Autodesk Inventor part; units mm, degrees
ref_plane "Work Plane1" through (-97.3094, -87.3563, -6.35) normal (0, 0, -1) x (0, 1, 0)
ref_plane "YZ Plane" through (0, 0, 0) normal (1, 0, 0) x (0, 1, 0)
ref_plane "XZ Plane" through (0, 0, 0) normal (0, 1, 0) x (-1, 0, 0)
sketch "Sketch1" plane through (0, 0, 0) normal (0, 0, 1) x (1, 0, 0)
  line L0 (-65.7194, 60.3542) -> (-75.7574, -47.1434)
  line L1 (-75.7574, -47.1434) -> (65.7194, -60.3542)
  line L2 (-95.8276, -262.0778) -> (45.6492, -275.2887)
  line L3 (-105.8656, -369.5754) -> (-95.8276, -262.0778)
  line L4 (-212.6955, 74.0786) -> (-222.7334, -33.419)
  line L5 (-222.7334, -33.419) -> (-364.2102, -20.2081)
  line L6 (-242.8036, -248.3534) -> (-384.2805, -235.1426)
  line L7 (-252.8416, -355.851) -> (-242.8036, -248.3534)
  circle A0 centre (-72.4386, -92.2695) radius 2.6 construction
  circle A1 centre (-84.3392, -219.7151) radius 2.6 construction
  circle A2 centre (3.2796, -227.8968) radius 2.6 construction
  circle A3 centre (15.1803, -100.4512) radius 2.6 construction
  circle A4 centre (-156.3158, -105.5656) radius 1.7526 construction
  circle A5 centre (-164.2553, -190.5905) radius 1.7526 construction
  circle A6 centre (-246.2503, -204.5961) radius 2.6 construction
  circle A7 centre (-333.8691, -196.4144) radius 2.6 construction
  circle A8 centre (-321.9685, -68.9688) radius 2.6 construction
  circle A9 centre (-234.3496, -77.1505) radius 2.6 construction
  circle A10 centre (15.1803, -100.4512) radius 1.6
  circle A11 centre (3.2796, -227.8968) radius 1.6
  circle A12 centre (-84.3392, -219.7151) radius 1.6
  circle A13 centre (-72.4386, -92.2695) radius 1.6
  circle A14 centre (-234.3496, -77.1505) radius 1.6
  circle A15 centre (-321.9685, -68.9688) radius 1.6
  circle A16 centre (-333.8691, -196.4144) radius 1.6
  circle A17 centre (-246.2503, -204.5961) radius 1.6
  line L8 (-65.7194, 60.3542) -> (-212.6955, 74.0786)
  line L9 (-364.2102, -20.2081) -> (-384.2805, -235.1426)
  line L10 (-252.8416, -355.851) -> (-105.8656, -369.5754)
  line L11 (45.6492, -275.2887) -> (65.7194, -60.3542)
  circle A18 centre (-156.3158, -105.5656) radius 1.8288
  circle A19 centre (-164.2553, -190.5905) radius 1.8288
  point P0 (0, 0)
  dimension "d0" = 3.2
  dimension "d1" = 3.2
  dimension "d2" = 3.2
  dimension "d3" = 3.2
  dimension "d4" = 3.2
  dimension "d5" = 3.2
  dimension "d6" = 3.2
  dimension "d7" = 3.2
  dimension "d8" = 3.6576
  dimension "d9" = 3.6576
ref_plane "Work Plane1" through (-97.3094, -87.3563, -6.35) normal (0, 0, -1) x (0, 1, 0)
extrude "Extrusion1" add sketch "Sketch1" against normal up to surface (6.35 mm away)
properties part number "Pod_Holders" material "Aluminum"
Can you work these out from the model? Positions are in its coordinate system, mm. A direction names the side the tool comes from. Give positions to 0.01 mm unless a question says otherwise; leave off trailing zeros. Loops run counter-clockwise (first coordinate to the right, second up) from the corner with the lowest first, then second, coordinate; pieces in that order, holes last. Notation, with made-up numbers: M 47.5,12 L 74.5,12 A14 ccw 74.5,25 Z; hole C -4,35 d2. An arc over 180 degrees is marked long. One line per item, written item: value.
1) Please list where these lines run through material, in increasing order: line 1 (X direction, y = -100, z = -4); line 2 (X direction, y = -218.5, z = -4.75); line 3 (X direction, y = 15.5, z = -3.5).
Geometry check:
line 1: x = -371.66 to 13.65, 16.72 to 62.02
line 2: x = -382.73 to -85.38, -83.3 to 50.95
line 3: x = -218.17 to -69.91
2) I'm going to push flat-ended pins straight in: pin 1 (4 mm diameter, centred on x = -321.97, y = -68.97, fed in from -Z); pin 2 (3 mm diameter, centred on x = -234.35, y = -77.15, fed in from -Z). Where does each tip first touch, or does it pass through?
Geometry check:
pin 1: stops at z = -6.35
pin 2: passes through
3) Imagine slicing it at C-C on x = -129. Write out the boundary of the cut face in (y, z).
Geometry check:
outline: M -367.42,-6.35 L 66.26,-6.35 L 66.26,0 L -367.42,0 Z
4) Imagine slicing it at B-B on y = -212. Write out the boundary of the cut face in (x, z).
Geometry check:
outline: M -382.12,-6.35 L 51.56,-6.35 L 51.56,0 L -382.12,0 Z
5) Thinking about a two-plate mould opening in X: for faces 1 (the face through (-374.105, -126.171, -3.131)), 2 (the face through (-292.481, -26.906, -3.131)), 3 (the face through (-70.668, 7.358, -3.131)), which applies, +X half, -X half, draft (parallel to the pull), parting line (faces both ways), or undercut?
Geometry check:
face 1: -X half
face 2: undercut
face 3: +X half
6) Imagine slicing it at A-A on z = -1.5. Count the separate pieces of the cut face and the enclosed holes in it, and give its area (3 significant figures).
Geometry check:
separate pieces: 1
enclosed holes: 10
area: 125,000 mm²
7) On a 3-axis mill with a long thin cutter (end or side, diameter ignored), from which of +Z, -Z, +X, -X, +Y, -Y can I reach the whole of each face in a straight line? I mean faces 4 (the face through (55.544, -169.326, -3.131)), 5 (the face through (-26.08, -268.59, -3.13)), 6 (the face through (-247.893, -302.855, -3.131)). Say none if no direction works.
Geometry check:
face 4: +Z, -Z, +X, -Y
face 5: +Z, -Z, -Y
face 6: +Z, -Z, -X
